Study the drawing (mm; zero at the part's minimum x, y, z) and answer. A direction names the side the tool comes from. Round coordinates to 2 decimals unless told otherwise and drop trailing zeros. Loops run counter-clockwise (first coordinate to the right, second up) from the corner with the lowest first, then second, coordinate; pieces in that order, holes last. Notation, with made-up numbers: M 70,41 L 80,41 A10 ccw 80,46 Z; hole C -33,72 d7. An arc over 180 degrees is marked long. Put each result on its own line as item: value. Start each with the question number.
(1) Straight lines are drawn through the part: line 1 (Z direction, x = 35, y = 29.5); line 2 (X direction, y = 20, z = 21); line 3 (X direction, y = 44, z = 29.5). For each, find the intervals that lie inside material, in ascending order.
(2) Determine the mould class of the marked faces 4, 5 and 6 for opening direction Y: released by +Y, released by -Y, zero draft, split by the parting line, or undercut.
(3) Which of the six approach directions +Z, -Z, +X, -X, +Y, -Y give full straight-line access (tool end or side, diameter ignored) to the marked faces 1, 2 and 3?
(4) Section B-B, the plane x = 15 is taken. Determine the outline of the cut face in (y, z).
(5) Section A-A, the plane y = 21.5 is taken. Determine the outline of the cut face in (x, z).
(6) Section D-D, the plane y = 16 is taken. Determine the outline of the cut face in (x, z).
(7) Section C-C, the plane z = 31 is taken. Determine the outline of the cut face in (x, y), then the cut area to 3 significant figures.
(8) Flat-ended cylindrical pins translate along their axes: P1, Ø15, axis at x = 43.5, y = 41.5, coming from the +Z side; P2, Ø5, axis at x = 48, y = 20, coming from the -Z side; P3, Ø8, axis at x = 39.5, z = 38, coming from the +Y side; P4, Ø5, axis at y = 44.5, z = 33, coming from the -X side. Find the tip coordinate at first contact, or state that the pin passes through.
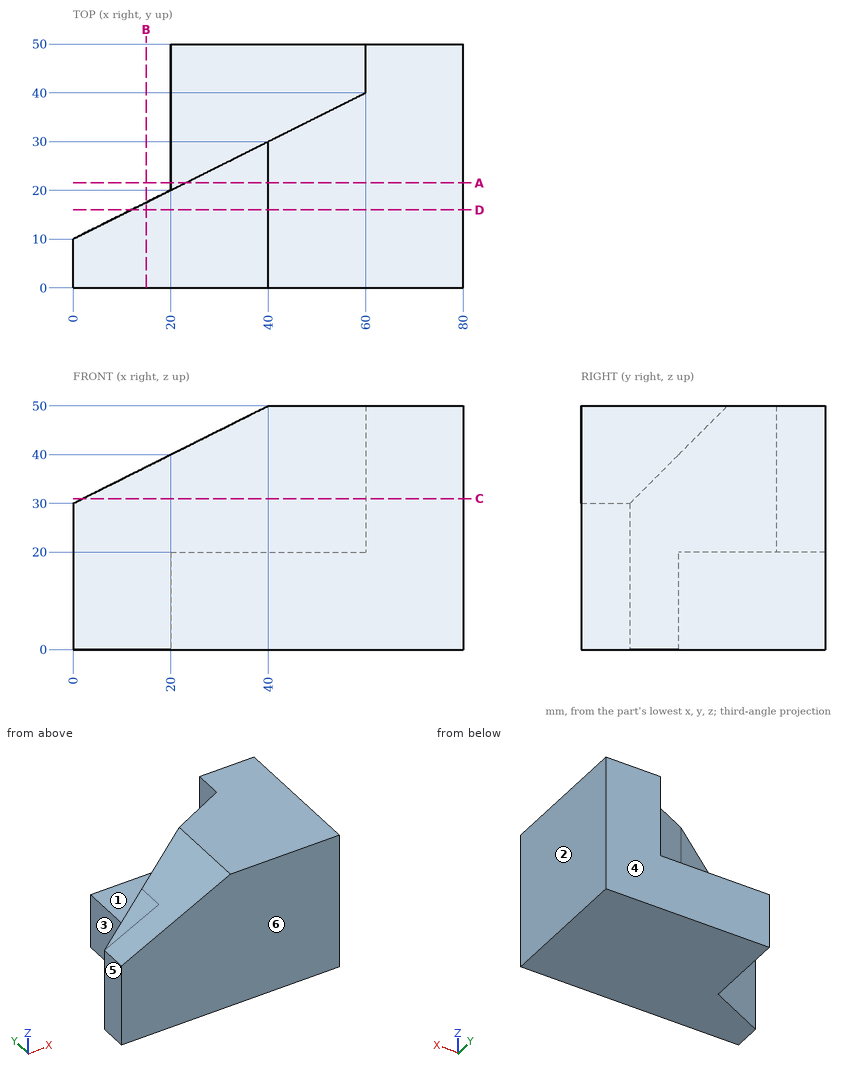
Recorded:
1. line 1: z = 0 to 20
1. line 2: x = 20 to 80
1. line 3: x = 60 to 80
2. face 4: released by +Y
2. face 5: zero draft
2. face 6: released by -Y
3. face 1: +Z, -X, +Y
3. face 2: +Z, -Z, +X, +Y, -Y
3. face 3: +Z, -Z, -X, +Y
4. outline: M 0,0 L 17.5,0 L 17.5,37.5 L 0,37.5 Z
5. outline: M 20,0 L 80,0 L 80,50 L 40,50 L 23,41.5 L 23,20 L 20,20 Z
6. outline: M 12,0 L 80,0 L 80,50 L 40,50 L 12,36 Z
7. outline: M 2,0 L 80,0 L 80,50 L 60,50 L 60,40 L 2,11 Z
7. area: 2,480 mm²
8. P1: stops at z = 20
8. P2: stops at z = 0
8. P3: stops at y = 31.75
8. P4: stops at x = 60
